Geometry check sheet. Reference: drawing and pictorial views, mm from the part's lowest x, y, z. Round coordinates to 2 decimals unless told otherwise and drop trailing zeros. Write each loop counter-clockwise with the first axis right and the second up, starting at its lowest first coordinate (ties: lowest second). Pieces come first, ordered by that corner, then holes. Notation, with made-up numbers: M 14,84 L 36,84 A24 cw 36,111 Z; hole C 16,-40 d9. An arc over 180 degrees is marked long. Answer in a Markdown table with one row per item.
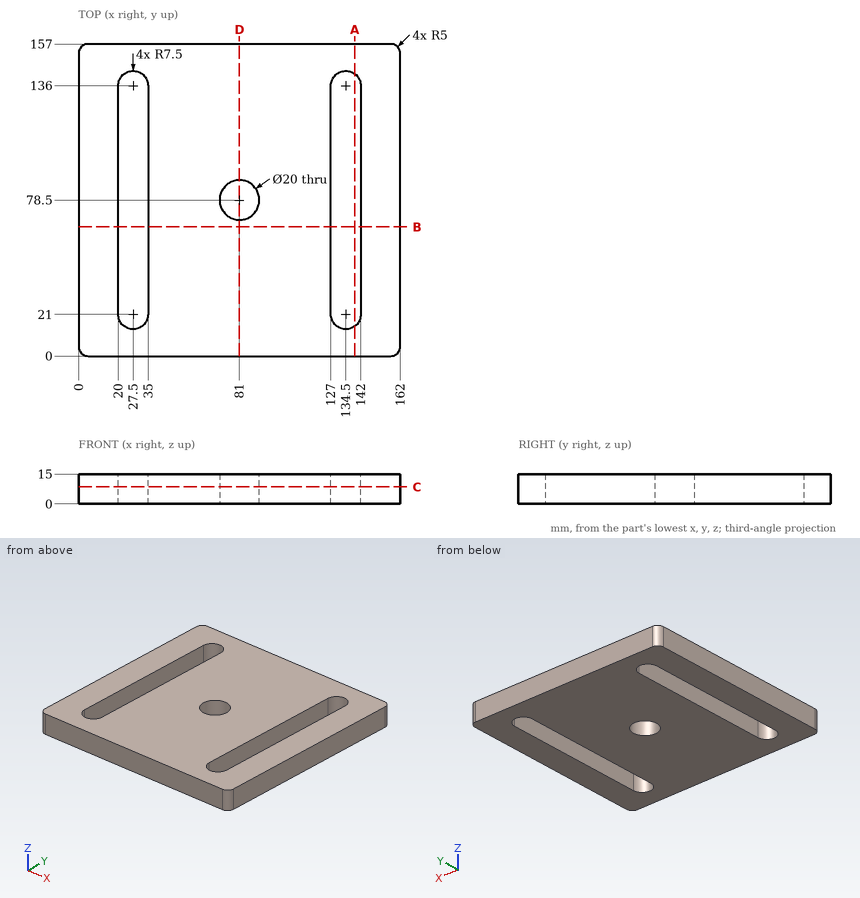
1. Section check A-A, the plane x = 139. Record the cut outline in (y, z), and give its area (3 significant figures).
Found:
| item | result |
|---|---|
| outline | M 0,0 L 15,0 L 15,15 L 0,15 Z; M 142,0 L 157,0 L 157,15 L 142,15 Z |
| area | 450 mm2 |
2. Section check C-C, the plane z = 8.5. Record the cut outline in (x, y), and give its area (3 significant figures).
Found:
| item | result |
|---|---|
| outline | M 0,5 A5 ccw 5,0 L 157,0 A5 ccw 162,5 L 162,152 A5 ccw 157,157 L 5,157 A5 ccw 0,152 Z; hole M 20,21 A7.5 ccw 35,21 L 35,136 A7.5 ccw 20,136 Z; hole C 81,78.5 d20; hole M 127,21 A7.5 ccw 142,21 L 142,136 A7.5 ccw 127,136 Z |
| area | 21,300 mm2 |
3. Section check D-D, the plane x = 81. Record the cut outline in (y, z).
Found:
| item | result |
|---|---|
| outline | M 0,0 L 68.5,0 L 68.5,15 L 0,15 Z; M 88.5,0 L 157,0 L 157,15 L 88.5,15 Z |
4. Section check B-B, the plane y = 65. Record the cut outline in (x, z), and give its area (3 significant figures).
Found:
| item | result |
|---|---|
| outline | M 0,0 L 20,0 L 20,15 L 0,15 Z; M 35,0 L 127,0 L 127,15 L 35,15 Z; M 142,0 L 162,0 L 162,15 L 142,15 Z |
| area | 1,980 mm2 |
5. Scan lines: L1, parallel to X at y = 106.5, z = 10.25; L2, parallel to Y at x = 81, z = 3.5; L3, parallel to Y at x = 134, z = 5.5. Record each from-to range of solid material in increasing order.
Found:
| item | result |
|---|---|
| L1 | x = 0 to 20, 35 to 127, 142 to 162 |
| L2 | y = 0 to 68.5, 88.5 to 157 |
| L3 | y = 0 to 13.52, 143.48 to 157 |
